Can you work these out from the model? Positions are in its coordinate system, mm. A direction names the side the tool comes from. Coordinates: 2 decimals unless noted, no trailing zeros. Write each loop counter-clockwise with the first axis right and the second up, starting at its lowest first coordinate (ties: lowest second). Pieces come first, ordered by that corner, then holes.
```python
from build123d import *

# Parameters (mm, degrees)
F1_DEPTH = 5
F2_W     = 5
F2_H     = 94
F3_DEPTH = 12
F5_DEPTH = 5


with BuildPart() as f1:
    # F0 (on Top) → F1 (new body)
    with BuildSketch(Plane.XY):
        Polygon((-8.5, -47), (8.5, -47), (8.5, 47), (3.75, 47), (1.25, 47), (-8.5, 47), align=None)
    extrude(amount=F1_DEPTH)

    # F2 (on face) → F3 (join)
    with BuildSketch(Plane.XY.offset(5)):
        with Locations((-6, 0)):
            Rectangle(F2_W, F2_H)
    extrude(amount=F3_DEPTH)

    # F4 (on face) → F5 (join)
    with BuildSketch(Plane.YZ.offset(-3.5)):
        Polygon((50.75, 13.5), (47, 12.25), (47, 9.75), (50.75, 8.5), align=None)
    extrude(amount=-F5_DEPTH)


solid = f1.part
```
1. If we section it at C-C, the plane y = 37: List the corners of the cut face in (x, z) for me, plus the area to 3 significant figures.
2. If we section it at A-A, the plane x = -5.5: List the corners of the cut face in (y, z) for me.
3. If we section it at D-D, the plane x = -1: List the corners of the cut face in (y, z) for me.
4. I'm going to push flat-ended pins straight in: P1, Ø4, axis at x = -6, z = 14, coming from the +Y side; P2, Ø1, axis at y = 26.5, z = 6, coming from the +X side; P3, Ø6, axis at x = 4.5, y = -15, coming from the +Z side. Where does each tip first touch, or does it pass through?
5. We'd pull the mould along Y, two halves only. Please class faces 5 (the face through (-6, 47, 15)), 6 (the face through (-4, -47, 6)), 7 (the face through (-3.5, 1, 11)): released by +Y, released by -Y, zero draft, split by the parting line, or undercut.
6. If I drill on L1, parallel to Z at x = 0.5, y = -38; L2, parallel to Y at x = -6.5, z = 6.25; L3, parallel to X at y = 37, z = 14, over which ranges is the centre line in solid material (lowest first)?
7. Which directions (+Z, -Z, +X, -X, +Y, -Y) give clear straight access to the entire face, cutting with the end or side of a thin tool? Please do faces 1 (the face through (2, 1, 5)), 2 (the face through (-8.5, 1, 8)), 3 (the face through (-5.965, 48.901, 12.884)), 4 (the face through (-5.965, 48.849, 9.134)).
8. If we section it at B-B, the plane z = 4: List the corners of the cut face in (x, y) for me, plus the area to 3 significant figures.
Answers:
1. outline: (-8.5, 0) - (8.5, 0) - (8.5, 5) - (-3.5, 5) - (-3.5, 17) - (-8.5, 17) - close
1. area: 145 mm2
2. outline: (-47, 0) - (47, 0) - (47, 9.75) - (50.75, 8.5) - (50.75, 13.5) - (47, 12.25) - (47, 17) - (-47, 17) - close
3. outline: (-47, 0) - (47, 0) - (47, 5) - (-47, 5) - close
4. P1: stops at y = 50.75
4. P2: stops at x = -3.5
4. P3: stops at z = 5
5. face 5: undercut
5. face 6: released by -Y
5. face 7: zero draft
6. L1: z = 0 to 5
6. L2: y = -47 to 47
6. L3: x = -8.5 to -3.5
7. face 1: +Z, +X, +Y, -Y
7. face 2: +Z, -Z, -X, +Y, -Y
7. face 3: +Z, +X, -X
7. face 4: -Z, +X, -X
8. outline: (-8.5, -47) - (8.5, -47) - (8.5, 47) - (-8.5, 47) - close
8. area: 1,600 mm2
